```python
from build123d import *

# Parameters (mm, degrees)
F0_W     = 38.1
F0_H     = 152.4
F0_R     = 6.35
F1_DEPTH = 3.302
F2_W     = 38.1
F2_H     = 5.8965822577
F3_DEPTH = 12.7
F5_DEPTH = 25.4


with BuildPart() as f1:
    # F0 (on Top) → F1 (new body)
    with BuildSketch(Plane.XY):
        Rectangle(F0_W, F0_H)
        with Locations((0, -48.2141543601)):
            Circle(F0_R, mode=Mode.SUBTRACT)
        with Locations((0, -21.6441029067)):
            Circle(F0_R, mode=Mode.SUBTRACT)
        with Locations((0, 4.9259485466)):
            Circle(F0_R, mode=Mode.SUBTRACT)
        with Locations((0, 31.496)):
            Circle(F0_R, mode=Mode.SUBTRACT)
        with Locations((0, 58.0660514534)):
            Circle(F0_R, mode=Mode.SUBTRACT)
    extrude(amount=F1_DEPTH)

    # F2 (on face) → F3 (join)
    with BuildSketch(Plane.XY.offset(3.302)):
        with Locations((0, 73.2517088711)):
            Rectangle(F2_W, F2_H)
        with Locations((0, -73.2517088711)):
            Rectangle(F2_W, F2_H)
    extrude(amount=F3_DEPTH)

    # F4 (on face) → F5 (cut)
    with BuildSketch(Plane.XY.offset(3.302)):
        with BuildLine():
            ThreePointArc((-19.05, 33.1740033209), (-10.0697438789, 36.8937471999), (-6.35, 45.8740033209))
            ThreePointArc((-6.35, 45.8740033209), (-10.0697438789, 54.854259442), (-19.05, 58.5740033209))
            Line((-19.05, 58.5740033209), (-19.05, 33.1740033209))
        make_face()
        with BuildLine():
            ThreePointArc((-6.35, 20.4740033209), (-10.0697438789, 29.454259442), (-19.05, 33.1740033209))
            Line((-19.05, 33.1740033209), (-19.05, 7.7740033209))
            ThreePointArc((-19.05, 7.7740033209), (-10.0697438789, 11.4937471999), (-6.35, 20.4740033209))
        make_face()
        with BuildLine():
            ThreePointArc((-6.35, -4.9259966791), (-10.0697438789, 4.054259442), (-19.05, 7.7740033209))
            Line((-19.05, 7.7740033209), (-19.05, -17.6259966791))
            ThreePointArc((-19.05, -17.6259966791), (-10.0697438789, -13.9062528001), (-6.35, -4.9259966791))
        make_face()
        with BuildLine():
            ThreePointArc((-6.35, -30.3259966791), (-10.0697438789, -21.345740558), (-19.05, -17.6259966791))
            Line((-19.05, -17.6259966791), (-19.05, -43.0259966791))
            ThreePointArc((-19.05, -43.0259966791), (-10.0697438789, -39.3062528001), (-6.35, -30.3259966791))
        make_face()
        with BuildLine():
            Line((19.05, 33.1740033209), (19.05, 58.5740033209))
            ThreePointArc((19.05, 58.5740033209), (6.35, 45.8740033209), (19.05, 33.1740033209))
        make_face()
        with BuildLine():
            ThreePointArc((-6.35, -55.7259966791), (-10.0697438789, -46.745740558), (-19.05, -43.0259966791))
            Line((-19.05, -43.0259966791), (-19.05, -68.4259966791))
            ThreePointArc((-19.05, -68.4259966791), (-10.0697438789, -64.7062528001), (-6.35, -55.7259966791))
        make_face()
        with BuildLine():
            Line((19.05, 7.7740033209), (19.05, 33.1740033209))
            ThreePointArc((19.05, 33.1740033209), (6.35, 20.4740033209), (19.05, 7.7740033209))
        make_face()
        with BuildLine():
            Line((19.05, -17.6259966791), (19.05, 7.7740033209))
            ThreePointArc((19.05, 7.7740033209), (6.35, -4.9259966791), (19.05, -17.6259966791))
        make_face()
        with BuildLine():
            Line((19.05, -43.0259966791), (19.05, -17.6259966791))
            ThreePointArc((19.05, -17.6259966791), (6.35, -30.3259966791), (19.05, -43.0259966791))
        make_face()
        with BuildLine():
            Line((19.05, -68.4259966791), (19.05, -43.0259966791))
            ThreePointArc((19.05, -43.0259966791), (6.35, -55.7259966791), (19.05, -68.4259966791))
        make_face()
    extrude(amount=-F5_DEPTH, mode=Mode.SUBTRACT)


solid = f1.part
```
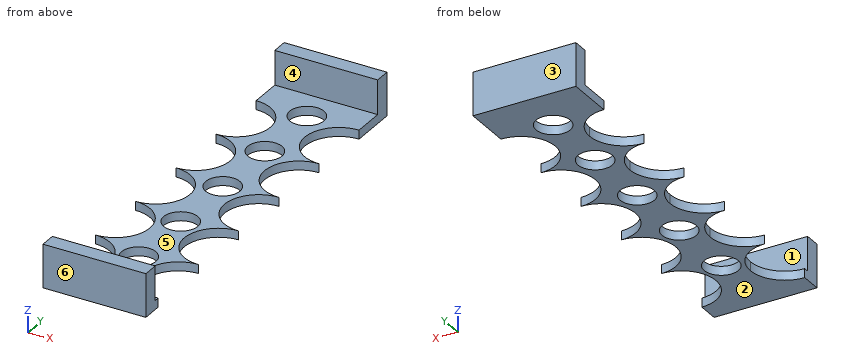
For this review, take the finished solid that the model builds, in its own axes (mm). Face numbers are marked on the shaded views. A direction names the side the tool comes from. Give positions to 0.01 mm unless a question says otherwise; leave off trailing zeros. Write each loop counter-clockwise with the first axis right and the second up, starting at its lowest first coordinate (ties: lowest second). Pieces come first, ordered by that corner, then holes. Notation, with made-up numbers: M 78.25,-34 L 114.25,-34 A25 ccw 114.25,-1 Z; hole C 57.25,-4 d3. An arc over 180 degrees is marked long. One line per item, written item: value.
1) For line 1 (Y direction, x = 0, z = 1); line 2 (Y direction, x = 17.5, z = 10.75); line 3 (Y direction, x = -9, z = 2), list the stretches that pass through material, from the lowest coordinate up. Write a range as from..to.
Results are:
line 1: y = -76.2..-54.56, -41.86..-27.99, -15.29..-1.42, 11.28..25.15, 37.85..51.72, 64.42..76.2
line 2: y = -76.2..-70.3, 70.3..76.2
line 3: y = -76.2..-63.49, -47.96..-38.09, -22.56..-12.69, 2.84..12.71, 28.24..38.11, 53.64..76.2
2) For P1, Ø7.5, axis at x = 0, y = 4.93, coming from the +Z side, flat-tipped, find the tip position at first contact; note if it passes through.
Results are:
P1: passes through
3) Take a section at A-A, the plane x = 0. Write out the cut boundary in (y, z), then the cut area to 3 significant figures.
Results are:
outline: M -76.2,0 L -54.56,0 L -54.56,3.3 L -70.3,3.3 L -70.3,16 L -76.2,16 Z; M -41.86,0 L -27.99,0 L -27.99,3.3 L -41.86,3.3 Z; M -15.29,0 L -1.42,0 L -1.42,3.3 L -15.29,3.3 Z; M 11.28,0 L 25.15,0 L 25.15,3.3 L 11.28,3.3 Z; M 37.85,0 L 51.72,0 L 51.72,3.3 L 37.85,3.3 Z; M 64.42,0 L 76.2,0 L 76.2,16 L 70.3,16 L 70.3,3.3 L 64.42,3.3 Z
area: 443 mm²
4) Take a section at C-C, the plane y = -23.5. Write out the cut boundary in (x, z), then the cut area to 3 significant figures.
Results are:
outline: M -8.34,0 L -6.07,0 L -6.07,3.3 L -8.34,3.3 Z; M 6.07,0 L 8.34,0 L 8.34,3.3 L 6.07,3.3 Z
area: 15.0 mm²
5) For the marked faces 5 and 6, list the 3-axis set-ups (+Z, -Z, +X, -X, +Y, -Y) from which the entire face can be reached by the end or side of a thin tool; tool diameter is ignored.
Results are:
face 5: +Z, +X, -X
face 6: +Z, -Z, +X, -X, -Y
6) The part is to be moulded in two halves that separate along Y. For the marked faces 1, 2, 3 and 4, say which applies: +Y half, -Y half, draft (parallel to the pull), parting line (faces both ways), or undercut.
Results are:
face 1: undercut
face 2: draft
face 3: +Y half
face 4: undercut
7) Take a section at D-D, the plane z = 1.75. Write out the cut boundary in (x, y), then the cut area to 3 significant figures.
Results are:
outline: M -19.05,-76.2 L 19.05,-76.2 L 19.05,-68.43 A12.7 cw 19.05,-43.03 A12.7 cw 19.05,-17.63 A12.7 cw 19.05,7.77 A12.7 cw 19.05,33.17 A12.7 cw 19.05,58.57 L 19.05,76.2 L -19.05,76.2 L -19.05,58.57 A12.7 cw -19.05,33.17 A12.7 cw -19.05,7.77 A12.7 cw -19.05,-17.63 A12.7 cw -19.05,-43.03 A12.7 cw -19.05,-68.43 Z; hole C 0,-48.21 d12.7; hole C 0,-21.64 d12.7; hole C 0,4.93 d12.7; hole C 0,31.5 d12.7; hole C 0,58.07 d12.7
area: 2,640 mm²
8) Take a section at B-B, the plane z = 11. Write out the cut boundary in (x, y).
Results are:
outline: M -19.05,-76.2 L 19.05,-76.2 L 19.05,-70.3 L -19.05,-70.3 Z; M -19.05,70.3 L 19.05,70.3 L 19.05,76.2 L -19.05,76.2 Z
